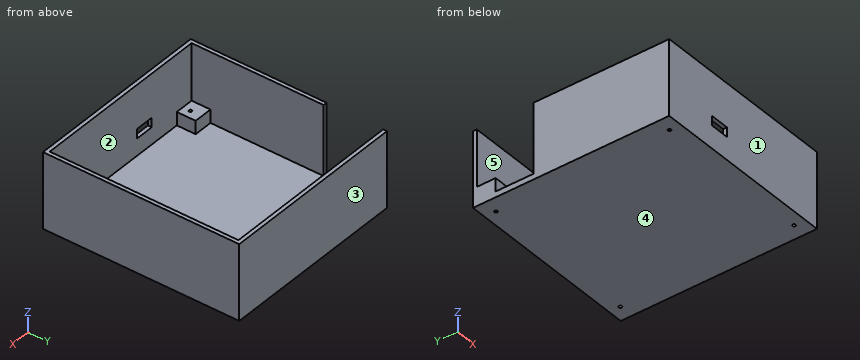
Autodesk Inventor part; units mm, degrees
ref_plane "YZ Plane" through (0, 0, 0) normal (1, 0, 0) x (0, 1, 0)
ref_plane "XZ Plane" through (0, 0, 0) normal (0, 1, 0) x (-1, 0, 0)
ref_plane "XY Plane" through (0, 0, 0) normal (0, 0, 1) x (1, 0, 0)
sketch "Sketch1" plane through (0, 0, 0) normal (0, 0, 1) x (1, 0, 0)
  line L0 (-65.4164, 28.1839) -> (34.5836, 28.1839)
  line L1 (34.5836, 28.1839) -> (34.5836, -75.8161)
  line L2 (34.5836, -75.8161) -> (-65.4164, -75.8161)
  line L3 (-65.4164, -75.8161) -> (-65.4164, 28.1839)
  point P0 (0, 0)
  dimension "d0" = 100
  dimension "d1" = 104
extrude "Extrusion1" add sketch "Sketch1" along normal blind 40
sketch "Sketch2" plane through (0, 0, 40) normal (0, 0, 1) x (1, 0, 0)
  line L0 (-63.4164, 26.1839) -> (32.5836, 26.1839)
  line L1 (32.5836, 26.1839) -> (32.5836, -73.8161)
  line L2 (32.5836, -73.8161) -> (-63.4164, -73.8161)
  line L3 (-63.4164, -73.8161) -> (-63.4164, 26.1839)
  line L4 (34.5836, 28.1839) -> (-65.4164, 28.1839)
  line L5 (34.5836, -75.8161) -> (34.5836, 28.1839)
  line L6 (-65.4164, 28.1839) -> (-65.4164, -75.8161)
  line L7 (-65.4164, -75.8161) -> (34.5836, -75.8161)
  point P0 (0, 0)
  dimension "d4" = 2
  dimension "d5" = 2
  dimension "d6" = 2
  dimension "d7" = 2
extrude "Extrusion2" cut sketch "Sketch2" against normal blind 37 contours L0 L1 L2 L3
sketch "Sketch3" plane through (0, 0, 3) normal (0, 0, 1) x (1, 0, 0)
  line L0 (-63.4164, 26.1839) -> (32.5836, 26.1839)
  line L1 (-63.4164, 26.1839) -> (-53.4164, 26.1839)
  line L2 (-53.4164, 26.1839) -> (-53.4164, 16.1839)
  line L3 (-53.4164, 16.1839) -> (-63.4164, 16.1839)
  line L4 (-63.4164, 16.1839) -> (-63.4164, 26.1839)
  line L5 (32.5836, 26.1839) -> (22.5836, 26.1839)
  line L6 (22.5836, 26.1839) -> (22.5836, 16.1839)
  line L7 (22.5836, 16.1839) -> (32.5836, 16.1839)
  line L8 (32.5836, 16.1839) -> (32.5836, 26.1839)
  line L9 (32.5836, -73.8161) -> (-63.4164, -73.8161)
  line L10 (-63.4164, -73.8161) -> (-53.4164, -73.8161)
  line L11 (-53.4164, -73.8161) -> (-53.4164, -63.8161)
  line L12 (-53.4164, -63.8161) -> (-63.4164, -63.8161)
  line L13 (-63.4164, -63.8161) -> (-63.4164, -73.8161)
  line L14 (32.5836, -73.8161) -> (22.5836, -73.8161)
  line L15 (22.5836, -73.8161) -> (22.5836, -63.8161)
  line L16 (22.5836, -63.8161) -> (32.5836, -63.8161)
  line L17 (32.5836, -63.8161) -> (32.5836, -73.8161)
  point P0 (0, 0)
  dimension "d10" = 10
  dimension "d11" = 10
  dimension "d12" = 10
  dimension "d13" = 10
  dimension "d14" = 10
  dimension "d15" = 10
  dimension "d16" = 10
  dimension "d17" = 10
extrude "Extrusion3" add sketch "Sketch3" along normal blind 7
sketch "Sketch4" plane through (0, 0, 40) normal (0, 0, 1) x (1, 0, 0)
  line L0 (-65.4164, 28.1839) -> (-65.4164, -75.8161)
  line L1 (-63.4164, 26.1839) -> (-65.4164, 26.1839)
  line L2 (-65.4164, 26.1839) -> (-65.4164, -3.8161)
  line L3 (-65.4164, -3.8161) -> (-63.4164, -3.8161)
  line L4 (-63.4164, -3.8161) -> (-63.4164, 26.1839)
  point P0 (0, 0)
  dimension "d20" = 30
extrude "Extrusion4" cut sketch "Sketch4" against normal up to surface (30 mm away)
sketch "Sketch5" plane through (0, 0, 10) normal (0, 0, 1) x (1, 0, 0)
  line L0 (-53.4164, 16.1839) -> (-63.4164, 16.1839)
  line L1 (-65.4164, 28.1839) -> (-65.4164, -75.8161)
  line L2 (-63.4164, 16.1839) -> (-65.4164, 16.1839)
  line L3 (-65.4164, 16.1839) -> (-65.4164, -3.8161)
  line L4 (-65.4164, -3.8161) -> (-63.4164, -3.8161)
  line L5 (-63.4164, -3.8161) -> (-63.4164, 16.1839)
  point P0 (0, 0)
  dimension "d23" = 20
extrude "Extrusion5" cut sketch "Sketch5" against normal up to surface (7 mm away)
sketch "Sketch6" plane through (0, 0, 10) normal (0, 0, 1) x (1, 0, 0)
  circle A0 centre (-57.5414, 22.1839) radius 0.8
  circle A1 centre (26.7086, 22.1839) radius 0.8
  circle A2 centre (26.7086, -69.8161) radius 0.8
  circle A3 centre (-57.5414, -69.8161) radius 0.8
  line L0 (32.5836, -73.8161) -> (-63.4164, -73.8161)
  line L1 (32.5836, 26.1839) -> (32.5836, -73.8161)
  line L2 (-63.4164, -73.8161) -> (-63.4164, -3.8161)
  line L3 (-65.4164, 26.1839) -> (32.5836, 26.1839)
  point P0 (0, 0)
  dimension "d26" = 1.6
  dimension "d27" = 1.6
  dimension "d28" = 1.6
  dimension "d29" = 1.6
  dimension "d30" = 4
  dimension "d31" = 5.875
  dimension "d32" = 4
  dimension "d33" = 5.875
  dimension "d34" = 5.875
  dimension "d35" = 5.875
  dimension "d36" = 4
  dimension "d37" = 4
extrude "Extrusion6" cut sketch "Sketch6" against normal through all
sketch "Sketch7" plane through (-63.4164, -73.8161, 40) normal (0, 1, 0) x (1, 0, 0)
  line L0 (27, 23) -> (37, 23)
  line L1 (37, 23) -> (37, 28)
  line L2 (37, 28) -> (27, 28)
  line L3 (27, 28) -> (27, 23)
  line L4 (0, 0) -> (0, 30)
  line L5 (86, 37) -> (10, 37)
  point P0 (63.4164, 40)
  dimension "d40" = 10
  dimension "d41" = 5
  dimension "d42" = 27
  dimension "d43" = 9
extrude "Extrusion7" cut sketch "Sketch7" against normal through all
properties part number "e_box"
The listing builds one solid part. Answer for the finished solid, in the listing's coordinates (mm). Face numbers are marked on the shaded views. A direction names the side the tool comes from. Coordinates: 2 decimals unless noted, no trailing zeros. Order: outer loops, then holes, each group sorted by start corner. A loop starts at its lowest first (then second) coordinate and runs counter-clockwise, first axis right, second up. Notation, with made-up numbers: (58.25, 69.5) -> (72.25, 69.5) arc R16 cw to (72.25, 74.5) -> close; hole circle Ø6 at (-40, 26). An arc over 180 degrees is marked (long way). Answer in a Markdown table with one row per item. Add a question column.
Item 1: Find section D-D (z = 35). Write down the section's boundary in (x, y), then the cut area to 3 significant figures.
Item 2: Each of these flat-tipped pins is pushed along its axis until it touches: P1, Ø8, axis at y = 15, z = 25, coming from the -X side; P2, Ø5, axis at x = -26, y = 10.5, coming from the +Z side; P3, Ø1.8, axis at x = -57.54, y = 22.18, coming from the +Z side. Where does it stop, or does it pass through?
Item 3: Find the intervals of material crossed by L1, parallel to X at y = -30.5, z = 9; L2, parallel to Y at x = -35.5, z = 10.5; L3, parallel to Z at x = -13.5, y = 6, in increasing order. Write a range as from..to.
Item 4: Find section A-A (z = 14). Write down the section's boundary in (x, y).
Item 5: Find section B-B (x = -32.5). Write down the section's boundary in (y, z), then the cut area to 3 significant figures.
Item 6: Determine the mould class of the marked faces 1, 2 and 3 for opening direction Y: +Y half, -Y half, draft (parallel to the pull), parting line (faces both ways), or undercut.
Item 7: Find section C-C (y = 17.5). Write down the section's boundary in (x, z), then the cut area to 3 significant figures.
Item 8: Which of the six approach directions +Z, -Z, +X, -X, +Y, -Y give full straight-line access (tool end or side, diameter ignored) to the marked faces 4 and 5?
Result set:
| question | item | result |
|---|---|---|
| 1 | outline | (-65.42, -75.82) -> (34.58, -75.82) -> (34.58, 28.18) -> (-65.42, 28.18) -> (-65.42, 26.18) -> (32.58, 26.18) -> (32.58, -73.82) -> (-63.42, -73.82) -> (-63.42, -3.82) -> (-65.42, -3.82) -> close |
| 1 | area | 740 mm² |
| 2 | P1 | stops at x = 32.58 |
| 2 | P2 | stops at z = 3 |
| 2 | P3 | stops at z = 10 |
| 3 | L1 | x = -65.42..-63.42, 32.58..34.58 |
| 3 | L2 | y = -75.82..-73.82, 26.18..28.18 |
| 3 | L3 | z = 0..3 |
| 4 | outline | (-65.42, -75.82) -> (-36.42, -75.82) -> (-36.42, -73.82) -> (-63.42, -73.82) -> (-63.42, -3.82) -> (-65.42, -3.82) -> close; (-65.42, 26.18) -> (32.58, 26.18) -> (32.58, -73.82) -> (-26.42, -73.82) -> (-26.42, -75.82) -> (34.58, -75.82) -> (34.58, 28.18) -> (-65.42, 28.18) -> close |
| 5 | outline | (-75.82, 0) -> (28.18, 0) -> (28.18, 40) -> (26.18, 40) -> (26.18, 3) -> (-73.82, 3) -> (-73.82, 12) -> (-75.82, 12) -> close; (-75.82, 17) -> (-73.82, 17) -> (-73.82, 40) -> (-75.82, 40) -> close |
| 5 | area | 450 mm² |
| 6 | face 1 | -Y half |
| 6 | face 2 | undercut |
| 6 | face 3 | +Y half |
| 7 | outline | (-65.42, 0) -> (34.58, 0) -> (34.58, 40) -> (32.58, 40) -> (32.58, 10) -> (22.58, 10) -> (22.58, 3) -> (-53.42, 3) -> (-53.42, 10) -> (-65.42, 10) -> close |
| 7 | area | 528 mm² |
| 8 | face 4 | -Z, +X, -X, +Y, -Y |
| 8 | face 5 | +Z |
